```python
from build123d import *

# Parameters (mm, degrees)
SKETCH1_W               = 1016
SKETCH1_H               = 50.8
BOSS_EXTRUDE1_DEPTH     = 6
CUT_EXTRUDE1_DEPTH      = 6
SKETCH3_R               = 14.097
CUT_EXTRUDE2_DEPTH      = 7
F_1_4_20_TAPPED_HOLE1_D = 5.1054
LPATTERN1_COUNT         = 16
LPATTERN1_PITCH         = 12.7
LPATTERN1_COUNT_DIR2    = 2
LPATTERN1_PITCH_DIR2    = 31.75
F_1_4_20_TAPPED_HOLE2_D = 5.1054


with BuildPart() as part:
    # Sketch1 → Boss-Extrude1 (new body)
    with BuildSketch(Plane(origin=(0, 0, 0), x_dir=(1, 0, 0), z_dir=(0, 1, 0))):
        with Locations((508, 25.4)):
            Rectangle(SKETCH1_W, SKETCH1_H)
    extrude(amount=BOSS_EXTRUDE1_DEPTH)

    # Sketch2 → Cut-Extrude1 (cut)
    with BuildSketch(Plane(origin=(0, 6, 0), x_dir=(1, 0, 0), z_dir=(0, 1, 0))):
        with BuildLine():
            Line((24.7, 29.9), (634.3, 29.9))
            ThreePointArc((634.3, 29.9), (638.8, 25.4), (634.3, 20.9))
            Line((634.3, 20.9), (24.7, 20.9))
            ThreePointArc((24.7, 20.9), (20.2, 25.4), (24.7, 29.9))
        make_face()
    extrude(amount=-CUT_EXTRUDE1_DEPTH, mode=Mode.SUBTRACT)

    # Sketch3 → Cut-Extrude2 (cut, through all)
    with BuildSketch(Plane(origin=(0, 6, 0), x_dir=(1, 0, 0), z_dir=(0, 1, 0))):
        with Locations((971.042, 25.4)):
            Circle(SKETCH3_R)
    extrude(amount=-CUT_EXTRUDE2_DEPTH, mode=Mode.SUBTRACT)

    # 1/4-20 Tapped Hole1 (through all)
    with Locations(Plane(origin=(0, 6, 0), x_dir=(1, 0, 0), z_dir=(0, 1, 0))):
        with Locations((25.4, 41.275)):
            f_1_4_20_tapped_hole1 = Hole(F_1_4_20_TAPPED_HOLE1_D / 2)

    # LPattern1: 1_4-20 Tapped Hole1 16 × 2
    with Locations(*[(i * LPATTERN1_PITCH, 0, j * LPATTERN1_PITCH_DIR2) for i in range(LPATTERN1_COUNT) for j in range(LPATTERN1_COUNT_DIR2) if (i, j) != (0, 0)]):
        add(f_1_4_20_tapped_hole1, mode=Mode.SUBTRACT)

    # 1/4-20 Tapped Hole2 (through all)
    with Locations(Plane(origin=(0, 6, 0), x_dir=(1, 0, 0), z_dir=(0, 1, 0))):
        with Locations((687.318420147, 38.490597432), (731.312510659, 13.090597432)):
            Hole(F_1_4_20_TAPPED_HOLE2_D / 2)


solid = part.part
```
Read the model definition and answer for the solid it produces. Units are mm, in the model's axes. Give positions to 0.01 mm unless a question says otherwise; leave off trailing zeros. Write each loop counter-clockwise with the first axis right and the second up, starting at its lowest first coordinate (ties: lowest second). Pieces come first, ordered by that corner, then holes. Notation, with made-up numbers: M 50.25,51 L 102.25,51 A33 ccw 102.25,82 Z; hole C 88.25,-2 d9. An arc over 180 degrees is marked long. Put each result on its own line as item: value. Start each with the question number.
1. Consider line 1 along Z through (x, y) = (177.8, 4.45); line 2 along X through (y, z) = (2.7, -25); line 3 along X through (y, z) = (4.55, -13). Determine where each line is inside the solid, lowest interval first.
2. The part is cut by section B-B, the plane y = 2.8. Give the number of separate pieces and of enclosed holes in the cut face, and give its area (3 significant figures).
3. The part is cut by section A-A, the plane x = 576.5. Give the vertices of the cut face in (y, z), and give its area (3 significant figures).
4. This flat-tipped pin is pushed along its axis until it touches: pin 1 Ø4.5 at (x, z) = (38.1, -9.525) entering from -Y. Where does it stop, or does it pass through?
Final values:
1. line 1: z = -50.8 to -43.83, -38.72 to -29.9, -20.9 to -12.08, -6.97 to 0
1. line 2: x = 0 to 20.22, 638.78 to 956.95, 985.13 to 1016
1. line 3: x = 0 to 728.76, 733.86 to 964.34, 977.75 to 1016
2. separate pieces: 1
2. enclosed holes: 36
2. area: 44,700 mm²
3. outline: M 0,-50.8 L 6,-50.8 L 6,-29.9 L 0,-29.9 Z; M 0,-20.9 L 6,-20.9 L 6,0 L 0,0 Z
3. area: 251 mm²
4. pin 1: passes through
